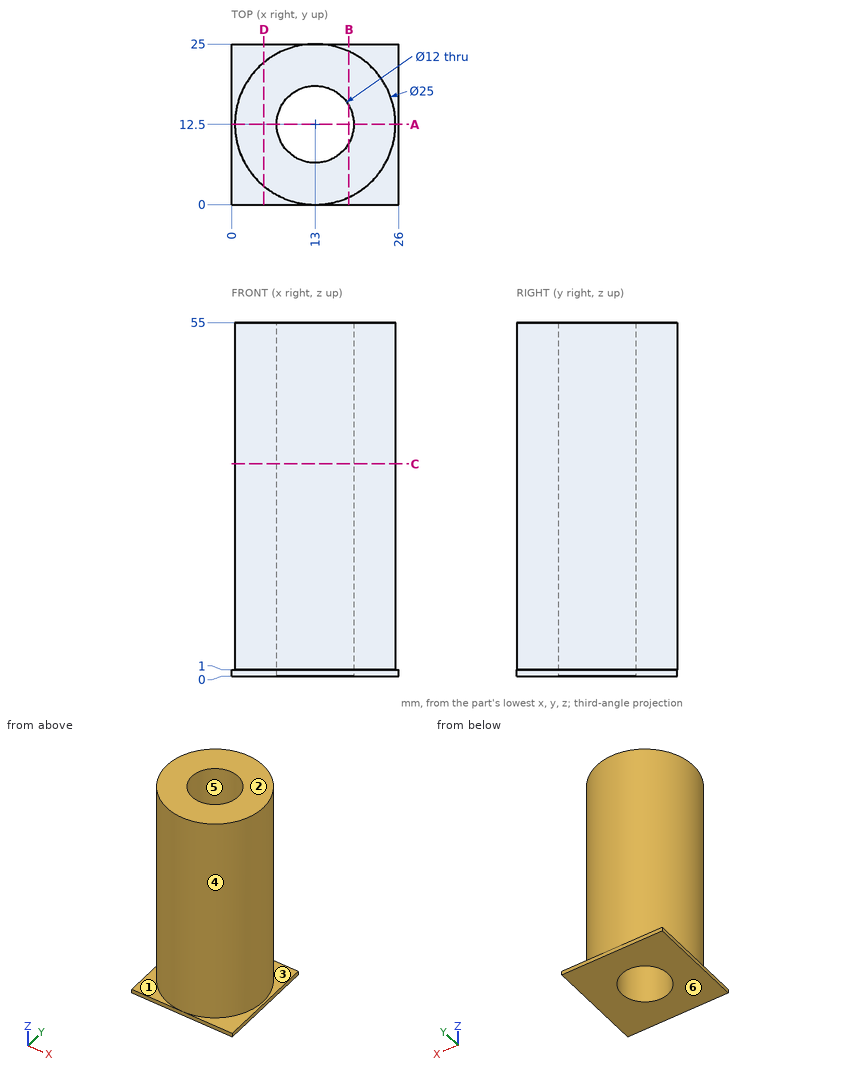
Geometry check sheet. Reference: drawing and pictorial views, mm from the part's lowest x, y, z. A direction names the side the tool comes from. Round coordinates to 2 decimals unless told otherwise and drop trailing zeros. Loops run counter-clockwise (first coordinate to the right, second up) from the corner with the lowest first, then second, coordinate; pieces in that order, holes last. Notation, with made-up numbers: (64.5, 1.5) - (99.5, 1.5) arc R24 cw to (99.5, 31.5) - close; hole circle Ø4 at (-18, -39.75). An arc over 180 degrees is marked (long way). Use a Markdown table: item, result.
Q1. Material ranges on line 1 (Y direction, x = 13, z = 13.5); line 2 (Z direction, x = 23, y = 4.75); line 3 (X direction, y = 14.5, z = 3), recorded low to high.
Solutions:
| item | result |
|---|---|
| line 1 | y = 0 to 6.5, 18.5 to 25 |
| line 2 | z = 0 to 1 |
| line 3 | x = 0.66 to 7.34, 18.66 to 25.34 |
Q2. Draft check along X on the marked faces 4, 5 and 6. Enter one of: released by +X, released by -X, zero draft, split by the parting line, or undercut.
Solutions:
| item | result |
|---|---|
| face 4 | split by the parting line |
| face 5 | undercut |
| face 6 | zero draft |
Q3. Cross-section at B-B on x = 18.25. Record the cut outline in (y, z), plus the area to 3 significant figures.
Solutions:
| item | result |
|---|---|
| outline | (0, 0) - (9.6, 0) - (9.6, 55) - (1.16, 55) - (1.16, 1) - (0, 1) - close; (15.4, 0) - (25, 0) - (25, 1) - (23.84, 1) - (23.84, 55) - (15.4, 55) - close |
| area | 931 mm2 |
Q4. Cross-section at C-C on z = 33. Record the cut outline in (x, y), plus the area to 3 significant figures.
Solutions:
| item | result |
|---|---|
| outline | circle Ø25 at (13, 12.5); hole circle Ø12 at (13, 12.5) |
| area | 378 mm2 |
Q5. Cross-section at A-A on y = 12.5. Record the cut outline in (x, z), plus the area to 3 significant figures.
Solutions:
| item | result |
|---|---|
| outline | (0, 0) - (7, 0) - (7, 55) - (0.5, 55) - (0.5, 1) - (0, 1) - close; (19, 0) - (26, 0) - (26, 1) - (25.5, 1) - (25.5, 55) - (19, 55) - close |
| area | 716 mm2 |
Q6. Cross-section at D-D on x = 5. Record the cut outline in (y, z), plus the area to 3 significant figures.
Solutions:
| item | result |
|---|---|
| outline | (0, 0) - (25, 0) - (25, 1) - (22.1, 1) - (22.1, 55) - (2.9, 55) - (2.9, 1) - (0, 1) - close |
| area | 1,060 mm2 |
Q7. Go/stop test with flat-tipped pins: P1, Ø12, axis at y = 13.5, z = 24, coming from the +X side; P2, Ø4, axis at y = 16, z = 41.5, coming from the -X side; P3, Ø8, axis at x = 17.5, z = 23, coming from the +Y side. Record where each tip stops, or that it passes through.
Solutions:
| item | result |
|---|---|
| P1 | stops at x = 25.5 |
| P2 | stops at x = 0.59 |
| P3 | stops at y = 24.99 |
Q8. Access from +Z, -Z, +X, -X, +Y, -Y to the whole of each face (thin tool, end or side, straight path). Record for the marked faces 1, 2 and 3.
Solutions:
| item | result |
|---|---|
| face 1 | +Z, -X |
| face 2 | +Z, +X, -X, +Y, -Y |
| face 3 | +Z, +X |
